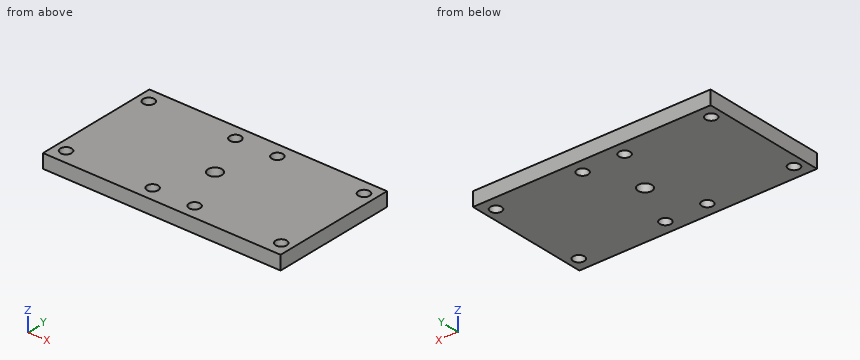
from build123d import *

# Parameters (mm, degrees)
SKETCH1_W                = 85
SKETCH1_H                = 45
BOSS_EXTRUDE1_DEPTH      = 5
CUT_EXTRUDE1_OUTLINE_R   = 2
CUT_EXTRUDE1_OUTLINE_R_2 = 2.5
CUT_EXTRUDE1_DEPTH       = 5


# Read off the part's stored shape, not the designer's step: Cut-Extrude1
with BuildPart() as part:
    # Sketch1 → Boss-Extrude1 (new body)
    with BuildSketch(Plane.XY):
        with Locations((-42.5, 22.5)):
            Rectangle(SKETCH1_W, SKETCH1_H)
    extrude(amount=BOSS_EXTRUDE1_DEPTH)

    # Cut-Extrude1 outline → Cut-Extrude1 (cut)
    with BuildSketch(Plane.XY):
        with Locations((-81, 40)):
            Circle(CUT_EXTRUDE1_OUTLINE_R)
        with Locations((-35, 5)):
            Circle(CUT_EXTRUDE1_OUTLINE_R)
        with Locations((-35, 40)):
            Circle(CUT_EXTRUDE1_OUTLINE_R)
        with Locations((-4, 40)):
            Circle(CUT_EXTRUDE1_OUTLINE_R)
        with Locations((-42.5, 22.5)):
            Circle(CUT_EXTRUDE1_OUTLINE_R_2)
        with Locations((-81, 5)):
            Circle(CUT_EXTRUDE1_OUTLINE_R)
        with Locations((-50, 5)):
            Circle(CUT_EXTRUDE1_OUTLINE_R)
        with Locations((-50, 40)):
            Circle(CUT_EXTRUDE1_OUTLINE_R)
        with Locations((-4, 5)):
            Circle(CUT_EXTRUDE1_OUTLINE_R)
    extrude(amount=CUT_EXTRUDE1_DEPTH, mode=Mode.SUBTRACT)


solid = part.part
Input: part model. Units: mm. Frame: model coordinates. Round coordinates to 2 decimals unless told otherwise and drop trailing zeros. Write each loop counter-clockwise with the first axis right and the second up, starting at its lowest first coordinate (ties: lowest second). Pieces come first, ordered by that corner, then holes.
1) Ray query, L1, parallel to Y at x = -35, z = 2.65; L2, parallel to Y at x = -42.5, z = 3.15; L3, parallel to X at y = 41, z = 2.5. Return the intervals inside material, ascending.
2) Contact query for a flat-ended pin moving along its axis: P1, Ø1, axis at x = -57.5, y = 18, coming from the -Z side. Output: stop coordinate, or through.
3) Cut plane A-A (x = -42.5). Return the cut outline in (y, z), then the cut area to 3 significant figures.
4) Cut plane B-B (y = 21). Return the cut outline in (x, z).
5) Cut plane D-D (x = -4). Return the cut outline in (y, z), then the cut area to 3 significant figures.
6) Cut plane C-C (z = 3.2). Count the separate pieces of the cut face and the enclosed holes in it, then the cut area to 3 significant figures.
Geometry says:
1. L1: y = 0 to 3, 7 to 38, 42 to 45
1. L2: y = 0 to 20, 25 to 45
1. L3: x = -85 to -82.73, -79.27 to -51.73, -48.27 to -36.73, -33.27 to -5.73, -2.27 to 0
2. P1: stops at z = 0
3. outline: (0, 0) - (20, 0) - (20, 5) - (0, 5) - close; (25, 0) - (45, 0) - (45, 5) - (25, 5) - close
3. area: 200 mm2
4. outline: (-85, 0) - (-44.5, 0) - (-44.5, 5) - (-85, 5) - close; (-40.5, 0) - (0, 0) - (0, 5) - (-40.5, 5) - close
5. outline: (0, 0) - (3, 0) - (3, 5) - (0, 5) - close; (7, 0) - (38, 0) - (38, 5) - (7, 5) - close; (42, 0) - (45, 0) - (45, 5) - (42, 5) - close
5. area: 185 mm2
6. separate pieces: 1
6. enclosed holes: 9
6. area: 3,700 mm2
